Autodesk Inventor part; units mm, degrees
ref_plane "YZ Plane" through (0, 0, 0) normal (1, 0, 0) x (0, 1, 0)
ref_plane "XZ Plane" through (0, 0, 0) normal (0, 1, 0) x (-1, 0, 0)
ref_plane "XY Plane" through (0, 0, 0) normal (0, 0, 1) x (1, 0, 0)
sketch "Sketch1" plane through (0, 0, 0) normal (0, 0, 1) x (1, 0, 0)
  line L0 (0, 0) -> (320, 0)
  line L1 (320, 0) -> (320, 16)
  line L2 (320, 16) -> (0, 16)
  line L3 (0, 16) -> (0, 0)
  line L4 (0, 0) -> (22.0483, 0)
  line L5 (10, 0) -> (29.5, 0)
  line L6 (29.5, 0) -> (29.5, -15)
  line L7 (29.5, -15) -> (10, -15)
  line L8 (10, -15) -> (10, 0)
  line L9 (308.4, 13.1) -> (311.6, 13.1)
  line L10 (311.6, 13.1) -> (311.6, 2.9)
  line L11 (311.6, 2.9) -> (308.4, 2.9)
  line L12 (308.4, 2.9) -> (308.4, 13.1)
  line L13 (308.4, 13.1) -> (311.6, 2.9) construction
  line L14 (311.6, 13.1) -> (308.4, 2.9) construction
  circle A0 centre (300, 11) radius 2.05
  circle A1 centre (290, 11) radius 2.05
  point P0 (0, 8)
  point P1 (310, 8)
  dimension "d2" = 19.5
  dimension "d3" = 15
  dimension "d4" = 10
  dimension "d5" = 16
  dimension "d8" = 320
  dimension "d13" = 10.2
  dimension "d14" = 3.2
  dimension "d15" = 10
  dimension "d16" = 4.1
  dimension "d18" = 4.1
  dimension "d20" = 10
  dimension "d21" = 20
  dimension "d23" = 5
extrude "Extrusion1" add sketch "Sketch1" along normal blind 3
sketch "Sketch2" plane through (0, 0, 3) normal (0, 0, 1) x (1, 0, 0)
  line L0 (0, 16) -> (0, 0)
  line L1 (0, 16) -> (0, 36)
  line L2 (320, 0) -> (320, 16)
  line L3 (320, 16) -> (320, 36)
  line L4 (320, 36) -> (0, 36)
  line L5 (320, 16) -> (0, 16)
  line L6 (50, 16) -> (50, 30)
  line L7 (50, 30) -> (210, 30)
  line L8 (210, 30) -> (210, 16)
  line L9 (40, 36) -> (36, 56)
  line L10 (36, 56) -> (42, 56)
  line L11 (42, 56) -> (46, 36)
  circle A0 centre (300, 11) radius 2.05
  line L12 (311.6, 13.1) -> (311.6, 2.9)
  circle A1 centre (310, 30) radius 2.1
  circle A2 centre (310, 20.6) radius 2.1
  point P0 (308.4, 13.1)
  point P1 (311.6, 8)
  dimension "d44" = 20
  dimension "d45" = 160
  dimension "d46" = 50
  dimension "d47" = 14
  dimension "d48" = 20
  dimension "d49" = 6
  dimension "d50" = 4
  dimension "d51" = 40
  dimension "d83" = 4.2
  dimension "d84" = 4.2
  dimension "d85" = 6
  dimension "d86" = 9.4
  dimension "d87" = 10
extrude "Extrusion2" add sketch "Sketch2" against normal blind 3 contours L1 L4 L3 L5 L8 L7 L6 | L9 L10 L11 L4
sketch "Sketch3" plane through (0, 0, 3) normal (0, 0, 1) x (1, 0, 0)
  circle A0 centre (16.5, -6.5) radius 2.1
  circle A1 centre (24.5, -7) radius 2.1
  line L0 (29.5, 0) -> (320, 0)
  line L1 (29.5, -15) -> (29.5, 0)
  point P0 (0, 0)
  dimension "d75" = 4.2
  dimension "d76" = 6.5
  dimension "d77" = 4.2
  dimension "d78" = 7
  dimension "d79" = 5
  dimension "d80" = 8
extrude "Extrusion3" cut sketch "Sketch3" against normal blind 3
sketch "Sketch4" plane through (0, 0, 3) normal (0, 0, 1) x (1, 0, 0)
  line L0 (39.9, 28.2) -> (45, 28.2)
  line L1 (45, 28.2) -> (45, 8)
  line L2 (45, 8) -> (39.9, 8)
  line L3 (39.9, 8) -> (39.9, 28.2)
  line L4 (50, 16) -> (50, 30)
  line L5 (29.5, 0) -> (320, 0)
  point P0 (0, 0)
  dimension "d88" = 5.1
  dimension "d89" = 20.2
  dimension "d90" = 5
  dimension "d91" = 8
extrude "Extrusion4" cut sketch "Sketch4" against normal blind 3
properties part number "Middle_bar"
Could you check a few things on this model? Use its own coordinates, in mm. Round coordinates to 2 decimals unless told otherwise and drop trailing zeros. Order: outer loops, then holes, each group sorted by start corner. A loop starts at its lowest first (then second) coordinate and runs counter-clockwise, first axis right, second up.
Q1. Please list where these lines run through material, in increasing order: probe 1 along Y at (x, z) = (310, 2.35); probe 2 along Y at (x, z) = (112.5, 2.65); probe 3 along Y at (x, z) = (16.5, 1.3).
Geometry says:
probe 1: y = 0 to 2.9, 13.1 to 18.5, 22.7 to 27.9, 32.1 to 36
probe 2: y = 0 to 16, 30 to 36
probe 3: y = -15 to -8.6, -4.4 to 36
Q2. I'm going to push flat-ended pins straight in: P1, Ø1.5, axis at x = 3.5, z = 2, coming from the -Y side; P2, Ø1.5, axis at y = 48, z = 2.5, coming from the +X side. Where does each tip first touch, or does it pass through?
Geometry says:
P1: stops at y = 0
P2: stops at x = 43.75
Q3. Imagine slicing it at C-C, the plane x = 216. List the corners of the cut face in (y, z) for me, then the cut area to 3 significant figures.
Geometry says:
outline: (0, 0) - (36, 0) - (36, 3) - (0, 3) - close
area: 108 mm2
Q4. Imagine slicing it at B-B, the plane x = 132.5. List the corners of the cut face in (y, z) for me, then the cut area to 3 significant figures.
Geometry says:
outline: (0, 0) - (16, 0) - (16, 3) - (0, 3) - close; (30, 0) - (36, 0) - (36, 3) - (30, 3) - close
area: 66.0 mm2
Q5. Imagine slicing it at A-A, the plane z = 1.85. State how many separate pieces and enclosed holes the cut face has, then the cut area to 4 significant figures.
Geometry says:
separate pieces: 1
enclosed holes: 9
area: 9,475 mm2
